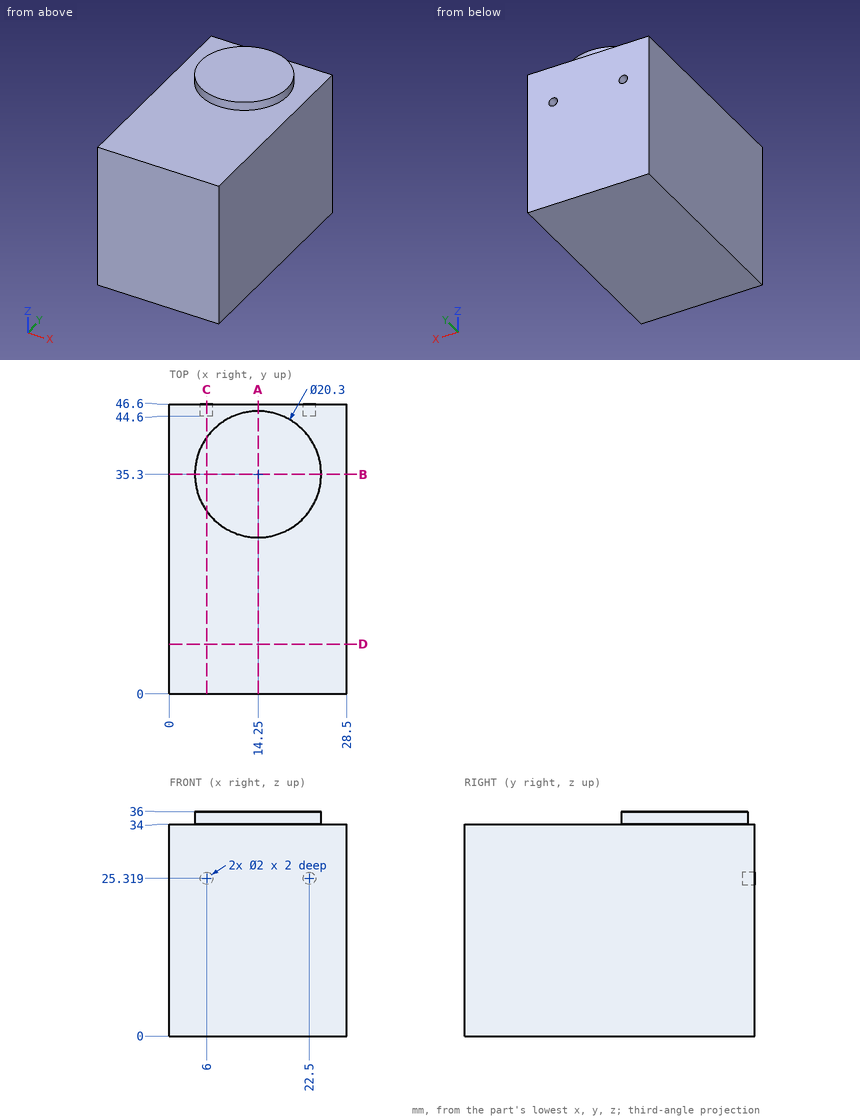
Geometry: see drawing. Coordinates: mm, zero at the bounding-box minimum. Round coordinates to 2 decimals unless told otherwise and drop trailing zeros. Loops run counter-clockwise (first coordinate to the right, second up) from the corner with the lowest first, then second, coordinate; pieces in that order, holes last. Notation, with made-up numbers: M 69.25,17 L 99.25,17 A29 cw 99.25,41 Z; hole C 64.5,-23 d2. An arc over 180 degrees is marked long. Use a Markdown table: item, result. Add a question column.
1. Contact query for flat-ended pins moving along their axis: pin 1 (8.5 mm diameter, centred on x = 7.5, y = 15, fed in from +Z); pin 2 (1.2 mm diameter, centred on x = 6, z = 25.32, fed in from +Y). Output: stop coordinate, or through.
2. Cut plane D-D, the plane y = 8. Output: boundary loops of the cut face in (x, z).
3. Cut plane C-C, the plane x = 6. Output: boundary loops of the cut face in (y, z).
4. Ray query, line 1 along Z through (x, y) = (4.5, 13). Return the intervals inside material, ascending. Write a range as [from, to].
5. Cut plane B-B, the plane y = 35.3. Output: boundary loops of the cut face in (x, z).
6. Cut plane A-A, the plane x = 14.25. Output: boundary loops of the cut face in (y, z).
Solution:
| question | item | result |
|---|---|---|
| 1 | pin 1 | stops at z = 34 |
| 1 | pin 2 | stops at y = 44.6 |
| 2 | outline | M 0,0 L 28.5,0 L 28.5,34 L 0,34 Z |
| 3 | outline | M 0,0 L 46.6,0 L 46.6,24.32 L 44.6,24.32 L 44.6,26.32 L 46.6,26.32 L 46.6,34 L 41.21,34 L 41.21,36 L 29.39,36 L 29.39,34 L 0,34 Z |
| 4 | line 1 | z = [0, 34] |
| 5 | outline | M 0,0 L 28.5,0 L 28.5,34 L 24.4,34 L 24.4,36 L 4.1,36 L 4.1,34 L 0,34 Z |
| 6 | outline | M 0,0 L 46.6,0 L 46.6,34 L 45.45,34 L 45.45,36 L 25.15,36 L 25.15,34 L 0,34 Z |
